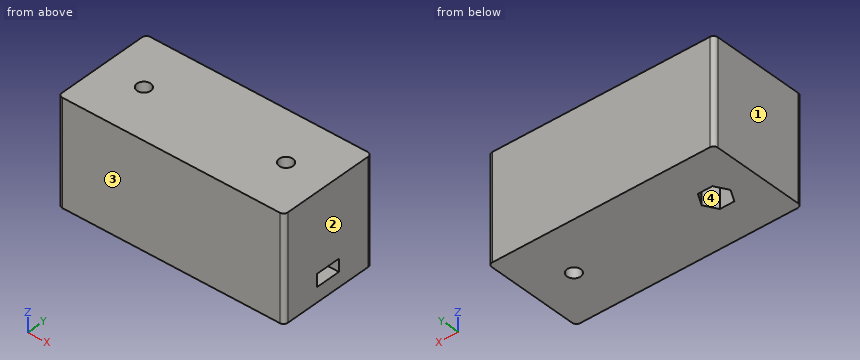
Solid Edge part; units mm, degrees
sketch "Sketch1" plane through (0, 0, 0) normal (0, 0, 1) x (1, 0, 0)
  line L0 (-27, -12) -> (27, -12)
  line L1 (27, -12) -> (27, 12)
  line L2 (27, 12) -> (-27, 12)
  line L3 (-27, 12) -> (-27, -12)
  dimension "D1" = 27
  dimension "D2" = 27
extrude "Ajout_matière_1" add sketch "Sketch1" along normal mid plane 25
fillet "Congé_1" radius 1 4 edges at (27, -12, 0) (27, 12, 0) (-27, -12, 0) (-27, 12, 0)
hole "Hole1" at (17, 0, 12.5) direction (0, 0, -1) diameter 3.3 end up to next
sketch "Sketch2" plane through (27, 0, 0) normal (1, 0, 0) x (0, 0, -1)
  line L0 (6, 3) -> (9, 3)
  line L1 (9, 3) -> (9, -3)
  line L2 (9, -3) -> (6, -3)
  line L3 (6, -3) -> (6, 3)
  dimension "D1" = 6
  dimension "D2" = 6
extrude "Enlèvement_matière_3" cut sketch "Sketch2" against normal blind 13.5
sketch "Sketch3" plane through (0, 0, -12.5) normal (0, 0, -1) x (0, 1, 0)
  line L0 (3, -15.2679) -> (0, -13.5359)
  line L1 (0, -13.5359) -> (-3, -15.2679)
  line L2 (-3, -15.2679) -> (-3, -18.7321)
  line L3 (-3, -18.7321) -> (0, -20.4641)
  line L4 (0, -20.4641) -> (3, -18.7321)
  line L5 (3, -18.7321) -> (3, -15.2679)
  dimension "D1" = 3
extrude "Cutout1" cut sketch "Sketch3" against normal blind 15
hole "Perçage_5" at (-17, 0, 2.5) direction (0, 0, 1) diameter 3.3 end up to next
properties material "Plastique ABS, haute performance"
The model under review builds one solid part; all positions refer to its coordinate system, in mm. Face numbers are marked on the shaded views. Give positions to 0.01 mm unless a question says otherwise; leave off trailing zeros. Write each loop counter-clockwise with the first axis right and the second up, starting at its lowest first coordinate (ties: lowest second). Pieces come first, ordered by that corner, then holes. Notation, with made-up numbers: (64.25, 21.25) - (114.25, 21.25) arc R17 ccw to (114.25, 48.25) - close; hole circle Ø9 at (14.25, 67). An arc over 180 degrees is marked (long way). Answer in a Markdown table with one row per item. Add a question column.
1. Insertion check: P1, Ø1.5, axis at y = -0.5, z = -8, coming from the +X side; P2, Ø2, axis at x = 17, y = 0, coming from the +Z side. Each pin has a flat end and moves straight along its axis. Give the tip position at first contact, or say it passes through.
2. We need section C-C on z = -1.75. Write out the cut boundary in (x, y), then the cut area to 3 significant figures.
3. We need section A-A on x = 17. Write out the cut boundary in (y, z), then the cut area to 3 significant figures.
4. We need section D-D on y = 0.75. Write out the cut boundary in (x, z).
5. Wall thickness on line 1 along X through (y, z) = (0, 4.75); line 2 along X through (y, z) = (0, -10.45); line 3 along Y through (x, z) = (17, 1.5): over which ranges is each line inside the solid? List them lowest first. Write a range as [from, to].
6. Draft analysis for pull direction X (two halves, no side actions). For the marked faces 1, 2, 3 and 4, state which applies: +X half, -X half, draft (parallel to the pull), parting line (faces both ways), or undercut.
7. We need section B-B on z = -8. Write out the cut boundary in (x, y).
Ans:
| question | item | result |
|---|---|---|
| 1 | P1 | stops at x = 13.5 |
| 1 | P2 | passes through |
| 2 | outline | (-27, -11) arc R1 ccw to (-26, -12) - (26, -12) arc R1 ccw to (27, -11) - (27, 11) arc R1 ccw to (26, 12) - (-26, 12) arc R1 ccw to (-27, 11) - close; hole (-20.46, 0) - (-18.73, -3) - (-15.27, -3) - (-13.54, 0) - (-15.27, 3) - (-18.73, 3) - close; hole circle Ø3.3 at (17, 0) |
| 2 | area | 1,260 mm^2 |
| 3 | outline | (-12, -12.5) - (-1.65, -12.5) - (-1.65, -9) - (-3, -9) - (-3, -6) - (-1.65, -6) - (-1.65, 12.5) - (-12, 12.5) - close; (1.65, -12.5) - (12, -12.5) - (12, 12.5) - (1.65, 12.5) - (1.65, -6) - (3, -6) - (3, -9) - (1.65, -9) - close |
| 3 | area | 509 mm^2 |
| 4 | outline | (-27, -12.5) - (-20.03, -12.5) - (-20.03, 2.5) - (-18.47, 2.5) - (-18.47, 12.5) - (-27, 12.5) - close; (-15.53, 2.5) - (-13.97, 2.5) - (-13.97, -12.5) - (15.53, -12.5) - (15.53, -9) - (13.5, -9) - (13.5, -6) - (15.53, -6) - (15.53, 12.5) - (-15.53, 12.5) - close; (18.47, -12.5) - (27, -12.5) - (27, -9) - (18.47, -9) - close; (18.47, -6) - (27, -6) - (27, 12.5) - (18.47, 12.5) - close |
| 5 | line 1 | x = [-27, -18.65], [-15.35, 15.35], [18.65, 27] |
| 5 | line 2 | x = [-27, -20.46], [-13.54, 15.35], [18.65, 27] |
| 5 | line 3 | y = [-12, -1.65], [1.65, 12] |
| 6 | face 1 | -X half |
| 6 | face 2 | +X half |
| 6 | face 3 | draft |
| 6 | face 4 | undercut |
| 7 | outline | (-27, -11) arc R1 ccw to (-26, -12) - (26, -12) arc R1 ccw to (27, -11) - (27, -3) - (13.5, -3) - (13.5, 3) - (27, 3) - (27, 11) arc R1 ccw to (26, 12) - (-26, 12) arc R1 ccw to (-27, 11) - close; hole (-20.46, 0) - (-18.73, -3) - (-15.27, -3) - (-13.54, 0) - (-15.27, 3) - (-18.73, 3) - close |
